from build123d import *

# Parameters (mm, degrees)
SKETCH_1_R               = 7.5
EXTRUDE_1_DEPTH          = 5
SKETCH_2_R               = 5
EXTRUDE_2_DEPTH          = 14
CUT_EXTRUDE_1_DEPTH      = 22.760055147
CUT_EXTRUDE_1_DEPTH_BACK = 3
SKETCH_3_W               = 2.708105792
SKETCH_3_H               = 12.424551298


with BuildPart() as part:
    # 草图1 → 凸台-拉伸1 (new body)
    with BuildSketch(Plane(origin=(0, 0, 0), x_dir=(1, 0, 0), z_dir=(0, 1, 0))):
        with Locations(Location((0, 0, 0), (0, 0, 270))):
            Circle(SKETCH_1_R)
    extrude(amount=EXTRUDE_1_DEPTH)

    # 草图2 → 凸台-拉伸2 (add)
    with BuildSketch(Plane(origin=(0, 0, 0), x_dir=(-1, 0, 0), z_dir=(0, -1, 0))):
        with Locations(Location((0, 0, 0), (0, 0, 90))):
            Circle(SKETCH_2_R)
    extrude(amount=EXTRUDE_2_DEPTH)

    # 草图3 → 切除-拉伸1 (cut, two sides: drawn at the far end of the back side and taken through both)
    with BuildSketch(Plane(origin=(0, 5, 0), x_dir=(1, 0, 0), z_dir=(0, 1, 0)).offset(-CUT_EXTRUDE_1_DEPTH_BACK)):
        Rectangle(SKETCH_3_W, SKETCH_3_H)
    extrude(amount=CUT_EXTRUDE_1_DEPTH + CUT_EXTRUDE_1_DEPTH_BACK, mode=Mode.SUBTRACT)


solid = part.part
Input: part model. Units: mm. Frame: model coordinates. A direction names the side the tool comes from. Coordinates: 2 decimals unless noted, no trailing zeros. Write each loop counter-clockwise with the first axis right and the second up, starting at its lowest first coordinate (ties: lowest second). Pieces come first, ordered by that corner, then holes. Notation, with made-up numbers: M -10,83 L 35,83 A29 ccw 35,114 Z; hole C 56,73 d8. An arc over 180 degrees is marked long. Answer as a JSON object with one key per item and string values. Group by question number.
(1) Set-up query: faces 1 (the face through (0.33, 2.465, -7.493)), 2 (the face through (0, 3, -6.212)), 3 (the face through (-5, 0, 2)). Return all of +Z, -Z, +X, -X, +Y, -Y with unobstructed straight access to the full face (end or side cutting, diameter ignored); none if empty.
(2) Ray query, line 1 along X through (y, z) = (3.25, 0.25); line 2 along Y through (x, z) = (-5, -2.75); line 3 along Y through (x, z) = (1.25, -2.5). Return the intervals inside material, ascending. Write a range as [from, to].
(3) Section A-A on y = 3.75. Output: boundary loops of the cut face in (x, z), plus the area to 3 significant figures.
(4) Section B-B on z = 0. Output: boundary loops of the cut face in (x, y), plus the area to 3 significant figures.
(5) Mould query, pull axis Z, two halves, no side actions, for faces 4 (the face through (-4.88, -6.9, 1.08)), 5 (the face through (0, 3, 6.212)), 6 (the face through (0, -14, 0)). Classes: pulls with the +Z half, pulls with the -Z half, needs draft (parallel to the pull), parting line crosses it, or undercut.
(6) Contact query for flat-ended pins moving along their axis: P1, Ø5, axis at x = 1, y = -3, coming from the +Z side; P2, Ø5, axis at y = -11, z = -0.5, coming from the -X side; P3, Ø1, axis at y = 0, z = 1.5, coming from the -X side. Output: stop coordinate, or through.
(7) Section C-C on x = 0. Output: boundary loops of the cut face in (y, z), plus the area to 3 significant figures.
(8) Section D-D on y = -3.5. Output: boundary loops of the cut face in (x, z), plus the area to 3 significant figures.
Result set:
{
 "1": {"face 1": "+Y, -Y", "face 2": "+Y", "face 3": "-Y"},
 "2": {"line 1": "x = [-7.5, -1.35], [1.35, 7.5]", "line 2": "y = [0, 5]", "line 3": "y = [-14, 2]"},
 "3": {"outline": "C 0,0 d15; hole M -1.35,-6.21 L 1.35,-6.21 L 1.35,6.21 L -1.35,6.21 Z", "area": "143 mm2"},
 "4": {"outline": "M -7.5,0 L -5,0 L -5,-14 L 5,-14 L 5,0 L 7.5,0 L 7.5,5 L 1.35,5 L 1.35,2 L -1.35,2 L -1.35,5 L -7.5,5 Z", "area": "207 mm2"},
 "5": {"face 4": "parting line crosses it", "face 5": "undercut", "face 6": "needs draft"},
 "6": {"P1": "stops at z = 5", "P2": "stops at x = -5", "P3": "stops at x = -7.43"},
 "7": {"outline": "M -14,-5 L 0,-5 L 0,-7.5 L 5,-7.5 L 5,-6.21 L 2,-6.21 L 2,6.21 L 5,6.21 L 5,7.5 L 0,7.5 L 0,5 L -14,5 Z", "area": "178 mm2"},
 "8": {"outline": "C 0,0 d10", "area": "78.5 mm2"}
}
